from build123d import *

# Parameters (mm, degrees)
CROQUIS1_R                   = 20
SALIENTE_EXTRUIR1_DEPTH      = 13.5
REDONDEO1_R                  = 2
CROQUIS2_W                   = 15.149467894
CROQUIS2_H                   = 37.020178586
SALIENTE_EXTRUIR2_DEPTH      = 26.39
SALIENTE_EXTRUIR3_DEPTH      = 5
SALIENTE_EXTRUIR3_DEPTH_BACK = 20.15
CROQUIS3_R                   = 4
REDONDEO2_R                  = 19


with BuildPart() as part:
    # Croquis1 → Saliente-Extruir1 (new body)
    with BuildSketch(Plane(origin=(0, 0, 0), x_dir=(1, 0, 0), z_dir=(0, 1, 0))):
        with Locations(Location((0, 0, 0), (0, 0, 270))):
            Circle(CROQUIS1_R)
    extrude(amount=SALIENTE_EXTRUIR1_DEPTH)

    # Redondeo1
    redondeo1_edges = [part.edges().sort_by_distance(p)[0] for p in [
        (0, 0, -20),
    ]]
    fillet(redondeo1_edges, radius=REDONDEO1_R)

    # Croquis2 → Saliente-Extruir2 (add)
    with BuildSketch(Plane(origin=(0, 13.5, 0), x_dir=(1, 0, 0), z_dir=(0, 1, 0))):
        Rectangle(CROQUIS2_W, CROQUIS2_H)
    extrude(amount=SALIENTE_EXTRUIR2_DEPTH)

    # Croquis3 → Saliente-Extruir3 (add, two sides: drawn at the far end of the back side and taken through both)
    with BuildSketch(Plane.ZY.offset(7.574733947).offset(-SALIENTE_EXTRUIR3_DEPTH_BACK)):
        with Locations((0, 27.11)):
            Circle(CROQUIS3_R)
    extrude(amount=SALIENTE_EXTRUIR3_DEPTH + SALIENTE_EXTRUIR3_DEPTH_BACK)

    # Redondeo2
    # the kernel refuses this fillet: 19 mm, written as the material it takes off along each edge
    with BuildSketch(Plane(origin=(55.074733947, 39.89, 18.510089293), x_dir=(0, -1, 0), z_dir=(-1, 0, 0)), Plane(origin=(-55.074733947, 39.89, -18.510089293), x_dir=(0, -1, 0), z_dir=(1, 0, 0))) as redondeo2_piece_1:
        with BuildLine():
            CenterArc((REDONDEO2_R, -REDONDEO2_R), REDONDEO2_R, 90, 90)
            Line((0, -REDONDEO2_R), (0, 0))
            Line((0, 0), (REDONDEO2_R, 0))
        make_face()
    extrude(amount=110.149467894, mode=Mode.SUBTRACT)


solid = part.part
Could you check a few things on this model? Use its own coordinates, in mm. A direction names the side the tool comes from. Coordinates: 2 decimals unless noted, no trailing zeros. Order: outer loops, then holes, each group sorted by start corner. A loop starts at its lowest first (then second) coordinate and runs counter-clockwise, first axis right, second up.
Q1. Will these pins go through, and if not, where does the flat tip stop? pin 1 (4 mm diameter, centred on x = -13.5, y = 23.5, fed in from -Z); pin 2 (2 mm diameter, centred on x = -2, y = 15.5, fed in from +Z); pin 3 (21 mm diameter, centred on y = 29.5, z = 0, fed in from -X).
Q2. Please list where these lines run through material, in increasing order: L1, parallel to X at y = 24, z = -9.5; L2, parallel to Y at x = -12, z = -12.5; L3, parallel to Y at x = 5, z = 4.
Q3. Which directions (+Z, -Z, +X, -X, +Y, -Y) give clear straight access to the entire face, cutting with the end or side of a thin tool? Please do faces 4 (the flat face through (-12.575, 27, 0)), 5 (the flat face through (0, 13.5, -19)), 6 (the flat face through (-12, 13.5, 0)), 7 (the flat face through (12, 13.5, 0)).
Q4. Suppose I cut it at D-D on y = 8.5. Please give me the cut outline in (x, z).
Q5. Suppose I cut it at B-B on y = 24.5. Please give me the cut outline in (x, z).
Q6. Suppose I cut it at A-A on x = 0. Please give me the cut outline in (y, z).
Q7. Thinking about a two-plate mould opening in Y: for faces 1 (the flat face through (0, 0, 0)), 2 (the cylindrical face through (-10.04, 31.076, -0.521)), 3 (the flat face through (0, 13.5, 19)), which applies, released by +Y, released by -Y, zero draft, split by the parting line, or undercut?
Q8. Suppose I cut it at C-C on y = 15. Please give me the cut outline in (x, z), and give its area (3 significant figures).
Answer:
1. pin 1: stops at z = -3.55
1. pin 2: stops at z = 18.51
1. pin 3: stops at x = -12.57
2. L1: x = -7.57 to 7.57
2. L2: y = 0 to 13.5
2. L3: y = 0 to 39.35
3. face 4: +Z, -Z, -X, +Y
3. face 5: -Z, +X, -X, +Y
3. face 6: +Z, -Z, -X
3. face 7: +Z, -Z, +X
4. outline: circle Ø40 at (0, 0)
5. outline: (-12.57, -3.03) - (-7.57, -3.03) - (-7.57, -18.16) - (7.57, -18.16) - (7.57, -3.03) - (12.58, -3.03) - (12.58, 3.03) - (7.57, 3.03) - (7.57, 18.16) - (-7.57, 18.16) - (-7.57, 3.03) - (-12.57, 3.03) - close
6. outline: (0, -18) arc R2 ccw to (2, -20) - (13.5, -20) - (13.5, -18.51) - (20.89, -18.51) arc R19 ccw to (39.88, 0) arc R19 ccw to (20.89, 18.51) - (13.5, 18.51) - (13.5, 20) - (2, 20) arc R2 ccw to (0, 18) - close
7. face 1: released by -Y
7. face 2: undercut
7. face 3: released by +Y
8. outline: (-7.57, -18.51) - (7.57, -18.51) - (7.57, 18.51) - (-7.57, 18.51) - close
8. area: 561 mm2
